Verification items for the finished model (mm, model axes). Round coordinates to 2 decimals unless told otherwise and drop trailing zeros. Loops run counter-clockwise (first coordinate to the right, second up) from the corner with the lowest first, then second, coordinate; pieces in that order, holes last. Notation, with made-up numbers: (31, 77.5) -> (86, 77.5) arc R22 ccw to (86, 86.5) -> close; hole circle Ø10 at (7, 79). An arc over 180 degrees is marked (long way). Write item = value, one per line.
Autodesk Inventor part; units mm, degrees
ref_plane "YZ Plane" through (0, 0, 0) normal (1, 0, 0) x (0, 1, 0)
ref_plane "XZ Plane" through (0, 0, 0) normal (0, 1, 0) x (-1, 0, 0)
ref_plane "XY Plane" through (0, 0, 0) normal (0, 0, 1) x (1, 0, 0)
sketch "Sketch1" plane through (0, 0, 0) normal (1, 0, 0) x (0, 1, 0)
  circle A0 centre (0, 0) radius 15.875
  line L0 (0, 0) -> (15.875, 0) construction
  circle A1 centre (9.525, 0) radius 1.7526
  circle A2 centre (0, 0) radius 9.525 construction
  circle A3 centre (0, 0) radius 5
  circle A4 centre (0, 9.525) radius 1.7526
  circle A5 centre (-9.525, 0) radius 1.7526
  circle A6 centre (0, -9.525) radius 1.7526
  dimension "d0" = 31.75
  dimension "d2" = 19.05
  dimension "d1" = 3.5052
  dimension "d3" = 10
  dimension "d6" = 360
extrude "Extrusion1" add sketch "Sketch1" along normal blind 3.175
chamfer "Chamfer1" distance 3.175 angle 45 4 edges at (0, 7.7724, 0) (0, -1.7526, -9.525) (0, -11.2776, 0) (0, -1.7526, 9.525)
properties part number "Spacer" material "UHMW, Black"
(1) Sectioned sample at A-A, the plane y = 0. Record the cut outline in (x, z) (3 decimals).
Filled sheet:
outline = (0, -15.875) -> (3.175, -15.875) -> (3.175, -11.278) -> (0, -14.453) -> close; (0, 14.453) -> (3.175, 11.278) -> (3.175, 15.875) -> (0, 15.875) -> close; (0.403, -5) -> (3.175, -7.772) -> (3.175, -5) -> close; (0.403, 5) -> (3.175, 5) -> (3.175, 7.772) -> close
(2) Material ranges on probe 1 along Y at (x, z) = (1.2, -3); probe 2 along Z at (x, y) = (1.45, 0) (3 decimals); probe 3 along Z at (x, y) = (0.45, 1.5), recorded low to high. Write a range as from..to.
Filled sheet:
probe_1 = -15.59..-11.74, -7.31..-4, 4..7.31, 11.74..15.59
probe_2 = -15.875..-13.003, -6.047..-5, 5..6.047, 13.003..15.875
probe_3 = -15.8..-13.74, -5.31..-4.77, 4.77..5.31, 13.74..15.8
(3) Go/stop test with a flat-tipped pin: pin 1 Ø1.5 at (x, z) = (2, 9.5) entering from -Y. Record where the tip stops, or that it passes through.
Filled sheet:
pin_1 = -13.25
(4) Sectioned sample at C-C, the plane x = 2.8. Record the cut outline in (y, z) (3 decimals).
Filled sheet:
outline = circle Ø31.75 at (0, 0); hole circle Ø4.255 at (-9.525, 0); hole circle Ø10 at (0, 0); hole circle Ø4.255 at (0, -9.525); hole circle Ø4.255 at (0, 9.525); hole circle Ø4.255 at (9.525, 0)
(5) Draft check along Z on faces 1 (the face through (2.976, -0.423, 11.43)), 2 (the face through (1.565, -3.441, 15.497)), 3 (the face through (3.175, -4, 4)). Enter one of: released by +Z, released by -Z, zero draft, split by the parting line, or undercut.
Filled sheet:
face_1 = undercut
face_2 = split by the parting line
face_3 = zero draft
